Here's how the part is built. I have some questions about the finished solid (model axes, mm). Face numbers are marked on the shaded views. A direction names the side the tool comes from. Coordinates: 2 decimals unless noted, no trailing zeros. Write each loop counter-clockwise with the first axis right and the second up, starting at its lowest first coordinate (ties: lowest second). Pieces come first, ordered by that corner, then holes.
(1) Please list where these lines run through material, in increasing order: probe 1 along X at (y, z) = (-13, 33); probe 2 along Z at (x, y) = (24, 0.5); probe 3 along Z at (x, y) = (-29, 23).
(2) For pin 1 Ø2 at (x, z) = (-17, 53) entering from -Y; pin 2 Ø12 at (x, y) = (22.5, 17.5) entering from +Z; pin 3 Ø6.5 at (x, y) = (-26.19, 26.19) entering from -Z; pin 4 Ø10 at (y, z) = (20, -4.5) entering from +X, each with a flat end and sliding along its axis, tell me the tip position at first contact or that it passes through.
(3) Imagine slicing it at D-D, the plane z = 18.5. List the corners of the cut face in (x, y) for me.
(4) Imagine slicing it at C-C, the plane x = -25. State how many separate pieces and enclosed holes the cut face has, plus the area to 3 significant figures.
(5) Which directions (+Z, -Z, +X, -X, +Y, -Y) give clear straight access to the entire face, cutting with the end or side of a thin tool? Please do the marked faces 1, 2, 3 and 4.
(6) Imagine slicing it at B-B, the plane z = 85.5. List the corners of the cut face in (x, y) for me, plus the area to 3 significant figures.
```python
from build123d import *

# Parameters (mm, degrees)
SKETCH1_R           = 28.448
EXTRUDE1_DEPTH      = 82.55
CUT_EXTRUDE1_DEPTH  = 34.1376
SKETCH13_W          = 10.541
SKETCH13_H          = 19.0627
S2D0011_W           = 5.4991
S2D0011_H           = 16.002
SKETCH16_W          = 76.2
SKETCH16_H          = 25.4
EXTRUDE2_DEPTH      = 31.75
EXTRUDE2_DEPTH_BACK = 31.75
SKETCH17_R          = 10.4775
CUT_EXTRUDE9_DEPTH  = 0.254
SKETCH18_R          = 10.4775
CUT_EXTRUDE10_DEPTH = 0.254
SKETCH21_R          = 6.9469
EXTRUDE3_DEPTH      = 1.27
CIRPATTERN2_COUNT   = 6
HOLE1_D             = 7.1374
HOLE1_DEPTH         = 25.4
CUT_EXTRUDE11_DEPTH = 3.175
CUT_EXTRUDE12_DEPTH = 4.0386


with BuildPart() as part:
    # Sketch1 → Extrude1 (new body)
    with BuildSketch(Plane.XY):
        Circle(SKETCH1_R)
    extrude(amount=EXTRUDE1_DEPTH)

    # Sketch2 → Cut-Extrude1 (cut, symmetric)
    with BuildSketch(Plane(origin=(0, 0, 0), x_dir=(0, 0, 1), z_dir=(1, 0, 0))):
        with BuildLine():
            Line((69.342, 28.448), (69.342, 25.781))
            ThreePointArc((69.342, 25.781), (69.490789755, 25.421789755), (69.85, 25.273))
            Line((69.85, 25.273), (82.55, 25.273))
            Line((82.55, 25.273), (82.55, 28.448))
            Line((82.55, 28.448), (69.342, 28.448))
        make_face()
    cut_extrude1 = extrude(amount=CUT_EXTRUDE1_DEPTH, both=True, mode=Mode.SUBTRACT)

    # Sketch10 → Cut-Revolve1 (revolve, cut)
    with BuildSketch(Plane(origin=(0, 0, 0), x_dir=(0, 0, -1), z_dir=(1, 0, 0)), mode=Mode.PRIVATE) as cut_revolve1_sk:
        Polygon((-82.55, 27.432), (-69.85, 27.432), (-68.834, 28.448), (-82.55, 28.448), align=None)
    revolve(cut_revolve1_sk.sketch.rotate(Axis((0, 0, 83.2358), (0, 0, -1)), 90), axis=Axis((0, 0, 83.2358), (0, 0, -1)), mode=Mode.SUBTRACT)  # turned: the seam where the file's is

    # Sketch13 → Revolve1 (revolve)
    with BuildSketch(Plane(origin=(0, 0, 0), x_dir=(0, 0, -1), z_dir=(1, 0, 0)), mode=Mode.PRIVATE) as revolve1_sk:
        with Locations((-87.8205, 9.53135)):
            Rectangle(SKETCH13_W, SKETCH13_H)
    revolve(revolve1_sk.sketch.rotate(Axis((0, 0, 93.61805), (0, 0, -1)), 90), axis=Axis((0, 0, 93.61805), (0, 0, -1)))  # turned: the seam where the file's is

    # S2D0011 → Cut-Revolve4 (revolve, cut)
    with BuildSketch(Plane(origin=(-5.4991, 0, 93.091), x_dir=(-1, 0, 0), z_dir=(0, 1, 0)), mode=Mode.PRIVATE) as cut_revolve4_sk:
        with Locations((-2.74955, -8.001)):
            Rectangle(S2D0011_W, S2D0011_H)
    revolve(cut_revolve4_sk.sketch.rotate(Axis((0, 0, 56.25285781), (0, 0, 1)), 180), axis=Axis((0, 0, 56.25285781), (0, 0, 1)), mode=Mode.SUBTRACT)  # turned: the seam where the file's is

    # Sketch15 → Cut-Revolve5 (revolve, cut)
    with BuildSketch(Plane(origin=(0, 0, 0), x_dir=(0, 0, -1), z_dir=(1, 0, 0)), mode=Mode.PRIVATE) as cut_revolve5_sk:
        with BuildLine():
            Line((-93.091, 14.2875), (-88.919964429, 18.809182473))
            ThreePointArc((-88.919964429, 18.809182473), (-88.65712697, 18.996541229), (-88.3412, 19.0627))
            Line((-88.3412, 19.0627), (-93.091, 19.0627))
            Line((-93.091, 19.0627), (-93.091, 14.2875))
        make_face()
    revolve(cut_revolve5_sk.sketch.rotate(Axis((0, 0, 93.32849), (0, 0, -1)), 90), axis=Axis((0, 0, 93.32849), (0, 0, -1)), mode=Mode.SUBTRACT)  # turned: the seam where the file's is

    # Sketch16 → Extrude2 (add, two sides)
    with BuildSketch(Plane(origin=(0, 0, 0), x_dir=(-1, 0, 0), z_dir=(0, 1, 0))) as extrude2_sk:
        with Locations((-6.35, 1.524)):
            Rectangle(SKETCH16_W, SKETCH16_H)
    extrude(amount=EXTRUDE2_DEPTH)
    extrude(extrude2_sk.sketch, amount=-EXTRUDE2_DEPTH_BACK)

    # Sketch17 → Cut-Extrude9 (cut)
    with BuildSketch(Plane(origin=(44.45, 0, 0), x_dir=(0, 0, -1), z_dir=(1, 0, 0))):
        with Locations((1.651, -15.875)):
            Circle(SKETCH17_R)
    extrude(amount=-CUT_EXTRUDE9_DEPTH, mode=Mode.SUBTRACT)

    # Sketch18 → Cut-Extrude10 (cut)
    with BuildSketch(Plane(origin=(44.45, 0, 0), x_dir=(0, 0, -1), z_dir=(1, 0, 0))):
        with Locations((1.651, 15.875)):
            Circle(SKETCH18_R)
    extrude(amount=-CUT_EXTRUDE10_DEPTH, mode=Mode.SUBTRACT)

    # S2D0002 → Cut-Revolve6 (revolve, cut)
    with BuildSketch(Plane(origin=(44.196, -15.875, -1.651), x_dir=(0, -1, 0), z_dir=(0, 0, 1)), mode=Mode.PRIVATE) as cut_revolve6_sk:
        Polygon((0, 0), (6.1849, 0), (5.642306865, -2.5527), (4.9784, -3.216606865), (4.9784, -17.272), (0, -17.272), align=None)
    revolve(cut_revolve6_sk.sketch.rotate(Axis((26.0604, -15.875, -1.651), (1, 0, 0)), 270), axis=Axis((26.0604, -15.875, -1.651), (1, 0, 0)), mode=Mode.SUBTRACT)  # turned: the seam where the file's is

    # S2D0001 → Cut-Revolve7 (revolve, cut)
    with BuildSketch(Plane(origin=(44.196, 15.875, -1.651), x_dir=(0, -1, 0), z_dir=(0, 0, 1)), mode=Mode.PRIVATE) as cut_revolve7_sk:
        Polygon((0, 0), (6.1849, 0), (5.642306865, -2.5527), (4.9784, -3.216606865), (4.9784, -17.272), (0, -17.272), align=None)
    revolve(cut_revolve7_sk.sketch.rotate(Axis((26.0604, 15.875, -1.651), (1, 0, 0)), 270), axis=Axis((26.0604, 15.875, -1.651), (1, 0, 0)), mode=Mode.SUBTRACT)  # turned: the seam where the file's is

    # Sketch21 → Extrude3 (add)
    with BuildSketch(Plane(origin=(44.196, 0, 0), x_dir=(0, 0, -1), z_dir=(1, 0, 0))):
        with Locations((1.651, -15.875)):
            Circle(SKETCH21_R)
    extrude(amount=EXTRUDE3_DEPTH)

    # CirPattern2: Cut-Extrude1 ×6 about axis
    cirpattern2_axis = Axis((0, 0, 0), (0, 0, 1))
    for i in range(1, CIRPATTERN2_COUNT):
        add(cut_extrude1.rotate(cirpattern2_axis, i * 360 / CIRPATTERN2_COUNT), mode=Mode.SUBTRACT)

    # Hole1
    with Locations(Plane.XY.offset(14.224)):
        with Locations((-26.1874, -26.1874), (34.925, 0), (-26.1874, 26.1874)):
            Hole(HOLE1_D / 2, depth=HOLE1_DEPTH)

    # Sketch24 → Cut-Revolve8 (revolve, cut)
    with BuildSketch(Plane(origin=(0, 0, 0), x_dir=(0, 0, -1), z_dir=(1, 0, 0)), mode=Mode.PRIVATE) as cut_revolve8_sk:
        Polygon((-93.091, 8.5344), (-92.2782, 9.3472), (-93.091, 10.16), align=None)
    revolve(cut_revolve8_sk.sketch.rotate(Axis((0, 0, 93.13164), (0, 0, -1)), 90), axis=Axis((0, 0, 93.13164), (0, 0, -1)), mode=Mode.SUBTRACT)  # turned: the seam where the file's is

    # Sketch25 → Cut-Extrude11 (cut)
    with BuildSketch(Plane.XY.offset(93.091)):
        with BuildLine():
            Line((-1.5875, 9.211405517), (-1.5875, -9.211405517))
            ThreePointArc((-1.5875, -9.211405517), (0, -9.3472), (1.5875, -9.211405517))
            Line((1.5875, -9.211405517), (1.5875, 9.211405517))
            ThreePointArc((1.5875, 9.211405517), (0, 9.3472), (-1.5875, 9.211405517))
        make_face()
    extrude(amount=-CUT_EXTRUDE11_DEPTH, mode=Mode.SUBTRACT)

    # Sketch26 → Cut-Extrude12 (cut)
    with BuildSketch(Plane.XY.offset(93.091)):
        with BuildLine():
            Line((-14.2875, 12.619582998), (-14.2875, -12.619582998))
            ThreePointArc((-14.2875, -12.619582998), (-19.0627, 0), (-14.2875, 12.619582998))
        make_face()
        with BuildLine():
            Line((14.2875, 12.619582998), (14.2875, -12.619582998))
            ThreePointArc((14.2875, -12.619582998), (19.0627, 0), (14.2875, 12.619582998))
        make_face()
    extrude(amount=-CUT_EXTRUDE12_DEPTH, mode=Mode.SUBTRACT)


solid = part.part
```
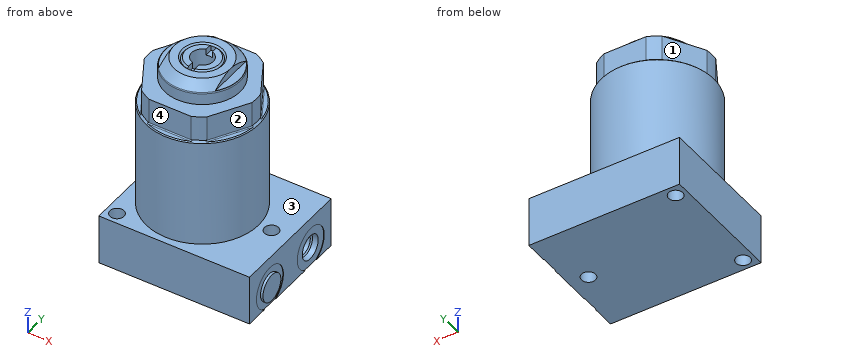
Recorded:
1. probe 1: x = -25.3 to 25.3
1. probe 2: z = -11.18 to 82.55
1. probe 3: z = -11.18 to 14.22
2. pin 1: stops at y = -23.52
2. pin 2: stops at z = 82.55
2. pin 3: passes through
2. pin 4: stops at x = 44.2
3. outline: circle Ø56.9 at (0, 0)
4. separate pieces: 3
4. enclosed holes: 0
4. area: 2,960 mm2
5. face 1: +Z, -X, +Y
5. face 2: +Z, +X, -Y
5. face 3: +Z
5. face 4: +Z, +X, -X, -Y
6. outline: circle Ø38.13 at (0, 0); hole circle Ø11 at (0, 0)
6. area: 1,050 mm2
